CAD build for the part. Positions are in the model's coordinates, mm. A direction names the side the tool comes from. Coordinates: 2 decimals unless noted, no trailing zeros. Loops run counter-clockwise (first coordinate to the right, second up) from the corner with the lowest first, then second, coordinate; pieces in that order, holes last.
1) Which spindle directions (+Z, -Z, +X, -X, +Y, -Y) get a long thin tool onto all of the face, cutting with end or side? Do faces 4 (the flat face through (2, 0, -17)), 5 (the cylindrical face through (-5.112, -5.07, -6.346)), 6 (the flat face through (2.1, -5, -1)). Say none if no direction does.
2) Saw through at A-A, the plane z = -33. Write the cut outline in (x, y), and give its area (3 significant figures).
3) Two-plate mould, pull along X, no slides. Class faces 1 (the flat face through (2, -10, -17)), 2 (the cylindrical face through (-0.572, -4.93, -10.092)), 3 (the cylindrical face through (-5.52, -4.93, -9.75)): +X half, -X half, draft (parallel to the pull), parting line (faces both ways), or undercut.
4) Pin check, flat tips, straight feed: pin 1 Ø1 at (x, y) = (-3.5, -4.5) entering from -Z; pin 2 Ø0.5 at (x, y) = (3, -5.5) entering from -Z; pin 3 Ø1.4 at (y, z) = (-7.5, -1) entering from -X. Stop position of each tip, or through.
5) Saw through at B-B, the plane x = -3.25. Give the number of separate pieces and of enclosed holes in the cut face, and give its area (3 significant figures).
6) Wall check: line 1 along Z through (x, y) = (5.5, -6.25); line 2 along Z through (x, y) = (-4, -6); line 3 along X through (y, z) = (-8.25, -29). Give the ranges that are in metal, low to high.
```python
from build123d import *

# Parameters (mm, degrees)
F1_DEPTH = 10
F2_R     = 1
F3_R     = 2
F4_R     = 0.5


with BuildPart() as f1:
    # F0 (on Front) → F1 (new body)
    with BuildSketch(Plane.XZ):
        with BuildLine():
            add(Edge.make_bspline(
                [(1.5112039039, 5.8065706541), (5.7834953099, 4.7065008724), (11.8156523878, -4.7347263591), (3.0061887209, -13.6750164571), (9.173676435, -21.061609973), (10.5198239377, -24.4136286822)],
                knots=[0.0047213261, 0.0047213261, 0.0047213261, 0.0047213261, 0.3509831279, 0.6641973473, 1, 1, 1, 1], degree=3))
            ThreePointArc((1.5112039039, 5.8065706541), (5.4017035076, 2.6118191391), (5.4896402552, -2.4215387398))
            ThreePointArc((5.4896402552, -2.4215387398), (6.2465875364, -3.188852596), (6.5231922366, -4.2305961251))
            ThreePointArc((6.5231922366, -4.2305961251), (6.225200021, -5.3089133071), (5.4157941938, -6.0812017975))
            ThreePointArc((5.4157941938, -6.0812017975), (3.0163538383, -12.9894945105), (-4.2289772618, -11.9960160364))
            add(Edge.make_bspline(
                [(-4.2289772618, -11.9960160364), (-2.1170324589, -14.4737038468), (1.871939821, -19.6061252586), (5.1872399636, -23.06487225), (6.4110226343, -25.9877145657)],
                knots=[0.0237271282, 0.0237271282, 0.0237271282, 0.0237271282, 0.5253023233, 1, 1, 1, 1], degree=3))
            ThreePointArc((6.4110226343, -25.9877145657), (-1.4294843622, -36.4738181218), (-7.5196663351, -24.8832356822))
            Line((-7.5196663351, -24.8832356822), (-11.3290949579, -22.6813619148))
            ThreePointArc((-11.3290949579, -22.6813619148), (-1.7772420469, -40.8600533084), (10.5198239377, -24.4136286822))
        make_face()
        with BuildLine():
            ThreePointArc((-1.7285399627, -1.1925391387), (-0.6245262518, 2.0049855263), (2.1, 0))
            Line((2.1, 0), (2.1, -2.3033259844))
            Line((2.1, -2.3033259844), (3.5891479903, -2.3033259844))
            ThreePointArc((3.5891479903, -2.3033259844), (4.5535626405, -2.1346468038), (5.4896402552, -2.4215387398))
            ThreePointArc((5.4896402552, -2.4215387398), (5.4017035076, 2.6118191391), (1.5112039039, 5.8065706541))
            ThreePointArc((1.5112039039, 5.8065706541), (1.4236796844, 5.8286478841), (1.3358332429, 5.849405914))
            ThreePointArc((1.3358332429, 5.849405914), (-4.6453170358, 3.7975030793), (-5.4670086667, -2.4722087772))
            Line((-5.4670086667, -2.4722087772), (-1.7285399627, -2.4722087772))
            Line((-1.7285399627, -2.4722087772), (-1.7285399627, -1.1925391387))
        make_face()
        with BuildLine():
            Line((3.4729907453, -6.1033259844), (2.1, -6.1033259844))
            Line((2.1, -6.1033259844), (2.1, -8.0709895119))
            ThreePointArc((2.1, -8.0709895119), (-0.6245262518, -10.0759750383), (-1.7285399627, -6.8784503732))
            Line((-1.7285399627, -6.8784503732), (-1.7285399627, -5.8205844834))
            Line((-1.7285399627, -5.8205844834), (-5.3127920255, -5.8205844834))
            ThreePointArc((-5.3127920255, -5.8205844834), (-5.7182347895, -8.8403222036), (-4.5291030542, -11.6455254849))
            add(Edge.make_bspline(
                [(-4.5291030542, -11.6455254849), (-4.4289292872, -11.7619570644), (-4.3288832889, -11.8788084534), (-4.2289772618, -11.9960160364)],
                knots=[0, 0, 0, 0, 0.0237271282, 0.0237271282, 0.0237271282, 0.0237271282], degree=3))
            ThreePointArc((-4.2289772618, -11.9960160364), (3.0163538383, -12.9894945105), (5.4157941938, -6.0812017975))
            ThreePointArc((5.4157941938, -6.0812017975), (4.4471049903, -6.3304599731), (3.4729907453, -6.1033259844))
        make_face()
    extrude(amount=F1_DEPTH)

    # F2
    f2_edges = [f1.edges().sort_by_distance(p)[0] for p in [
        (-1.72854, -5, -2.472209),
        (-1.72854, -5, -5.820584),
    ]]
    fillet(f2_edges, radius=F2_R)

    # F3
    f3_edges = [f1.edges().sort_by_distance(p)[0] for p in [
        (-11.329095, -5, -22.681362),
        (-7.519666, -5, -24.883236),
        (-5.467009, -5, -2.472209),
        (-5.312792, -5, -5.820584),
    ]]
    fillet(f3_edges, radius=F3_R)

    # F4
    f4_edges = [f1.edges().sort_by_distance(p)[0] for p in [
        (2.1, -5, -2.303326),
        (2.1, -5, -6.103326),
    ]]
    fillet(f4_edges, radius=F4_R)


solid = f1.part
```
Data:
1. face 4: +Z, -Z, +X, -X, +Y
1. face 5: -X, +Y, -Y
1. face 6: +Y, -Y
2. outline: (-12.19, -10) - (-7.29, -10) - (-7.29, 0) - (-12.19, 0) - close; (5.66, -10) - (10.56, -10) - (10.56, 0) - (5.66, 0) - close
2. area: 98.0 mm2
3. face 1: draft
3. face 2: undercut
3. face 3: -X half
4. pin 1: stops at z = -40.7
4. pin 2: stops at z = -40.36
4. pin 3: stops at x = -5.99
5. separate pieces: 3
5. enclosed holes: 0
5. area: 194 mm2
6. line 1: z = -39.12 to -33.23, -24.13 to -6.03, -2.43 to 3.44
6. line 2: z = -40.47 to -35.81, -12.27 to -5.83, -2.47 to 4.47
6. line 3: x = -12.96 to -8.55, 6.92 to 11.32
